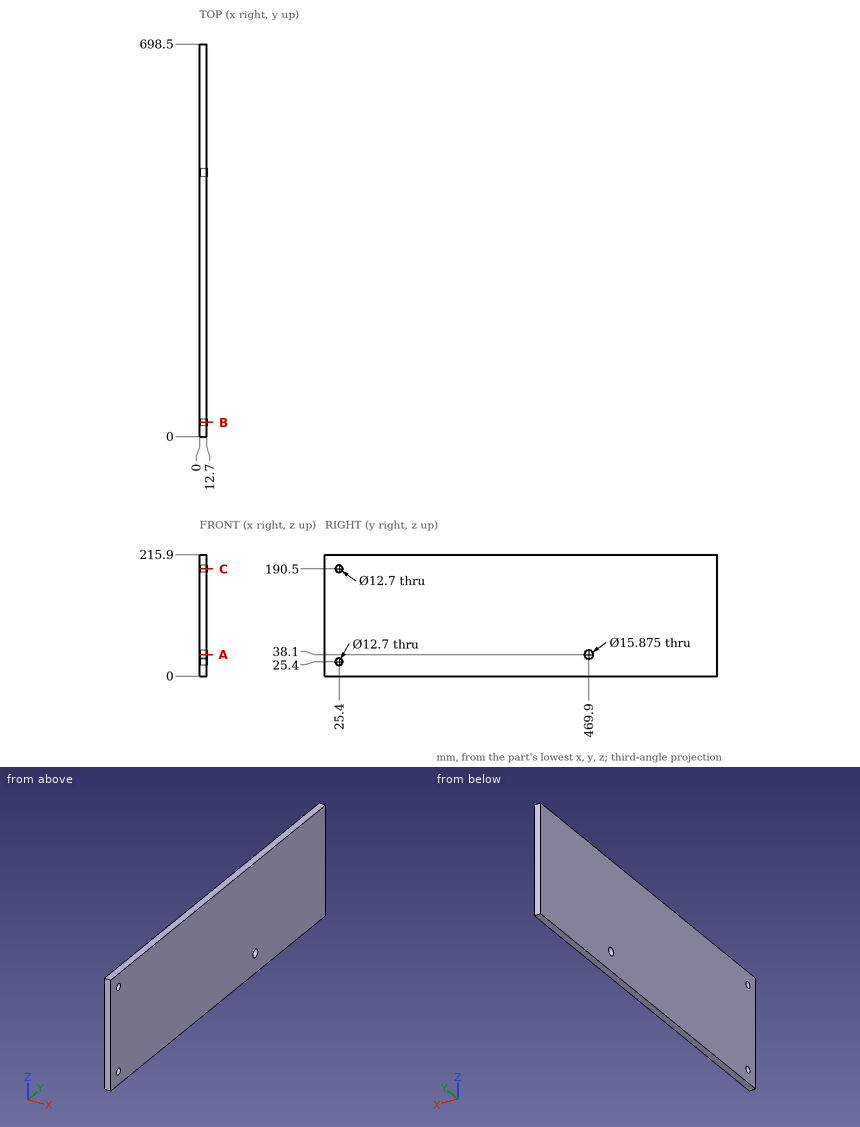
Here's the drawing with two shaded views (mm, measured from the low corner). I have some questions. Give positions to 0.01 mm unless a question says otherwise; leave off trailing zeros. Loops run counter-clockwise (first coordinate to the right, second up) from the corner with the lowest first, then second, coordinate; pieces in that order, holes last. Notation, with made-up numbers: M 49,37.5 L 79,37.5 A18 ccw 79,44.5 Z; hole C -19,29.5 d9. An arc over 180 degrees is marked long. Use one line per item in the form item = value. Start each with the question number.
(1) I want a section at C-C, the plane z = 190.5. Write out the boundary of the cut face in (x, y).
(2) I want a section at A-A, the plane z = 38.1. Write out the boundary of the cut face in (x, y).
(3) I'm going to push a flat-ended pin straight in: P1, Ø5, axis at x = 10.5, y = 486.5, coming from the -Z side. Where does the tip first touch, or does it pass through?
(4) Please list where these lines run through material, in increasing order: line 1 (Z direction, x = 6.25, y = 25.4); line 2 (Y direction, x = 2, z = 189.5); line 3 (Z direction, x = 6.75, y = 470.5).
(5) I want a section at B-B, the plane y = 25.4. Write out the boundary of the cut face in (x, z).
Worked out:
q1.outline = M 0,0 L 12.7,0 L 12.7,19.05 L 0,19.05 Z; M 0,31.75 L 12.7,31.75 L 12.7,698.5 L 0,698.5 Z
q2.outline = M 0,0 L 12.7,0 L 12.7,461.96 L 0,461.96 Z; M 0,477.84 L 12.7,477.84 L 12.7,698.5 L 0,698.5 Z
q3.P1 = 0
q4.line_1 = 0 to 19.05, 31.75 to 184.15, 196.85 to 215.9
q4.line_2 = 0 to 19.13, 31.67 to 698.5
q4.line_3 = 0 to 30.19, 46.01 to 215.9
q5.outline = M 0,0 L 12.7,0 L 12.7,19.05 L 0,19.05 Z; M 0,31.75 L 12.7,31.75 L 12.7,184.15 L 0,184.15 Z; M 0,196.85 L 12.7,196.85 L 12.7,215.9 L 0,215.9 Z
